Could you check a few things on this model? Use its own coordinates, in mm. Face numbers are marked on the shaded views. A direction names the side the tool comes from. Give positions to 0.01 mm unless a question says otherwise; leave off trailing zeros. Loops run counter-clockwise (first coordinate to the right, second up) from the corner with the lowest first, then second, coordinate; pieces in that order, holes last. Notation, with made-up numbers: (-31.5, 11.25) - (-19.5, 11.25) arc R21 ccw to (-19.5, 23.25) - close; hole circle Ø3 at (85.5, 32). An arc over 180 degrees is marked (long way). One line per item, written item: value. Start each with the question number.
Q1. I want a section at C-C (y = -26). Please give me the cut outline in (x, z), then the cut area to 3 significant figures.
Q2. I'm going to push flat-ended pins straight in: P1, Ø0.8, axis at x = 3.5, z = 9.5, coming from the -Y side; P2, Ø1.2, axis at x = -17, z = 18, coming from the -Y side; P3, Ø17, axis at x = 21.5, y = -12, coming from the +Z side. Where does each tip first touch, or does it pass through?
Q3. If I drill on line 1 (X direction, y = -20.5, z = 17.5); line 2 (Y direction, x = 3.5, z = 9.75); line 3 (Z direction, x = -26.5, y = -9), over which ranges is the centre line in solid material (lowest first)? Write a range as from..to.
Q4. I want a section at B-B (y = 20). Please give me the cut outline in (x, z).
Q5. If we mould it in two halves opening along Y, with no side actions, what happens to the marked faces 3, 4 and 5? For each: released by +Y, released by -Y, zero draft, split by the parting line, or undercut.
Q6. For the marked faces 1 and 2, which set-ups out of +Z, -Z, +X, -X, +Y, -Y let a thin tool reach every point of the face, with its end or its side?
```python
from build123d import *

# Parameters (mm, degrees)
F1_DEPTH = 20
F2_DEPTH = 5
F3_W     = 95
F3_H     = 1.5
F4_DEPTH = 0.75
F5_R     = 1
F6_DEPTH = 25


with BuildPart() as f1:
    # F0 (on Top) → F1 (new body)
    with BuildSketch(Plane.XY):
        with BuildLine():
            Line((-45, -30), (45, -30))
            ThreePointArc((45, -30), (48.535534, -28.535534), (50, -25))
            Line((50, -25), (50, 25))
            ThreePointArc((50, 25), (48.535534, 28.535534), (45, 30))
            Line((45, 30), (-45, 30))
            ThreePointArc((-45, 30), (-48.535534, 28.535534), (-50, 25))
            Line((-50, 25), (-50, -25))
            ThreePointArc((-50, -25), (-48.535534, -28.535534), (-45, -30))
        make_face()
        with BuildLine():
            ThreePointArc((-48, 23.32691), (-46.535534, 26.862444), (-43, 28.32691))
            Line((-43, 28.32691), (43, 28.32691))
            ThreePointArc((43, 28.32691), (46.535534, 26.862444), (48, 23.32691))
            Line((48, 23.32691), (48, -23.32691))
            ThreePointArc((48, -23.32691), (46.535534, -26.862444), (43, -28.32691))
            Line((43, -28.32691), (-43, -28.32691))
            ThreePointArc((-43, -28.32691), (-46.535534, -26.862444), (-48, -23.32691))
            Line((-48, -23.32691), (-48, 23.32691))
        make_face(mode=Mode.SUBTRACT)
    extrude(amount=F1_DEPTH)

    # F0 (on Top) → F2 (join)
    with BuildSketch(Plane.XY):
        with BuildLine():
            Line((43, 28.32691), (-43, 28.32691))
            ThreePointArc((-43, 28.32691), (-46.535534, 26.862444), (-48, 23.32691))
            Line((-48, 23.32691), (-48, -23.32691))
            ThreePointArc((-48, -23.32691), (-46.535534, -26.862444), (-43, -28.32691))
            Line((-43, -28.32691), (43, -28.32691))
            ThreePointArc((43, -28.32691), (46.535534, -26.862444), (48, -23.32691))
            Line((48, -23.32691), (48, 23.32691))
            ThreePointArc((48, 23.32691), (46.535534, 26.862444), (43, 28.32691))
        make_face()
    extrude(amount=F2_DEPTH)

    # F3 (on face) → F4 (cut)
    with BuildSketch(Plane.XZ.offset(30)):
        with Locations((0, 3.196598)):
            Rectangle(F3_W, F3_H)
        with Locations((0, 6.196598)):
            Rectangle(F3_W, F3_H)
        with Locations((0, 9.196598)):
            Rectangle(F3_W, F3_H)
        with Locations((0, 12.196598)):
            Rectangle(F3_W, F3_H)
        with Locations((0, 15.196598)):
            Rectangle(F3_W, F3_H)
        with Locations((0, 18.196598)):
            Rectangle(F3_W, F3_H)
    extrude(amount=-F4_DEPTH, mode=Mode.SUBTRACT)

    # F5 (on face) → F6 (cut)
    with BuildSketch(Plane.XZ.offset(-28.32691)):
        with Locations((-40.428117, 7.180942)):
            Circle(F5_R)
    extrude(amount=-F6_DEPTH, mode=Mode.SUBTRACT)


solid = f1.part
```
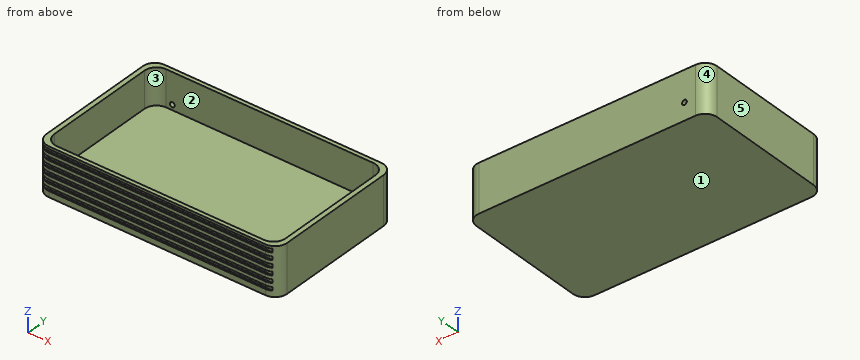
Worked answers:
1. outline: (-49.9, 0) - (49.9, 0) - (49.9, 20) - (47.23, 20) - (47.23, 5) - (-47.23, 5) - (-47.23, 20) - (-49.9, 20) - close
1. area: 579 mm²
2. P1: stops at y = -29.25
2. P2: stops at y = -30
2. P3: stops at z = 5
3. line 1: x = -50..-48, 48..50
3. line 2: y = -29.25..-28.33, 28.33..30
3. line 3: z = 0..5
4. outline: (-50, 0) - (50, 0) - (50, 20) - (48, 20) - (48, 5) - (-48, 5) - (-48, 20) - (-50, 20) - close
5. face 3: undercut
5. face 4: released by +Y
5. face 5: zero draft
6. face 1: -Z, +X, -X, +Y, -Y
6. face 2: +Z
